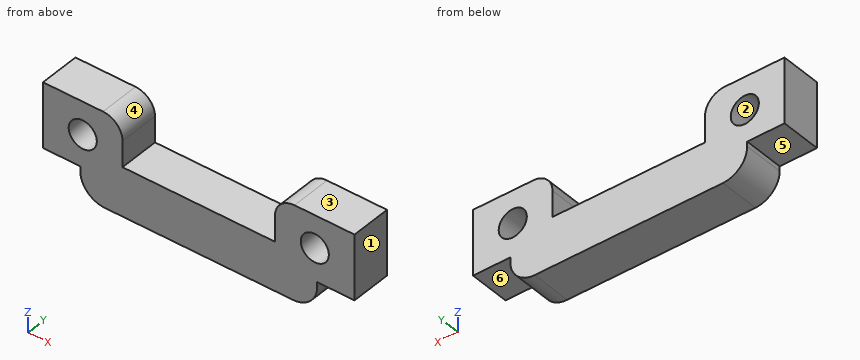
```python
from build123d import *

# Parameters (mm, degrees)
BOSS_EXTRUDE1_DEPTH  = 3.175
M2_CLEARANCE_HOLE1_D = 2.2
SKETCH4_W            = 2.921
SKETCH4_H            = 2.286
CUT_EXTRUDE1_DEPTH   = 4.175
FILLET1_R            = 1.905


with BuildPart() as part:
    # Sketch1 → Boss-Extrude1 (new body)
    with BuildSketch(Plane(origin=(0, 0, 0), x_dir=(1, 0, 0), z_dir=(0, 1, 0))):
        with BuildLine():
            Line((0, -0.127190553), (4.699, -0.127190553))
            ThreePointArc((4.699, -0.127190553), (5.776630735, 0.319178713), (6.223, 1.396809447))
            Line((6.223, 1.396809447), (6.223, 3.428809447))
            Line((6.223, 3.428809447), (18.161, 3.428809447))
            Line((18.161, 3.428809447), (18.161, 1.396809447))
            ThreePointArc((18.161, 1.396809447), (18.607369265, 0.319178713), (19.685, -0.127190553))
            Line((19.685, -0.127190553), (24.384, -0.127190553))
            Line((24.384, -0.127190553), (24.384, 7.238809447))
            Line((24.384, 7.238809447), (0, 7.238809447))
            Line((0, 7.238809447), (0, -0.127190553))
        make_face()
    extrude(amount=BOSS_EXTRUDE1_DEPTH)

    # M2 Clearance Hole1 (through all)
    with Locations(Plane(origin=(0, 0, 0), x_dir=(-1, 0, 0), z_dir=(0, -1, 0))):
        with Locations((-3.1115, 2.412809447), (-21.2725, 2.412809447)):
            Hole(M2_CLEARANCE_HOLE1_D / 2)

    # Sketch4 → Cut-Extrude1 (cut, through all)
    with BuildSketch(Plane.XZ):
        with Locations((22.9235, -6.095809447)):
            Rectangle(SKETCH4_W, SKETCH4_H)
        with Locations((1.4605, -6.095809447)):
            Rectangle(SKETCH4_W, SKETCH4_H)
    extrude(amount=-CUT_EXTRUDE1_DEPTH, mode=Mode.SUBTRACT)

    # Fillet1
    fillet1_edges = [part.edges().sort_by_distance(p)[0] for p in [
        (21.463, 1.5875, -7.238809447),
        (2.921, 1.5875, -7.238809447),
    ]]
    fillet(fillet1_edges, radius=FILLET1_R)


solid = part.part
```
Work out the finished part from the listing and answer in its coordinate system (mm). Face numbers are marked on the shaded views. A direction names the side the tool comes from. Coordinates: 2 decimals unless noted, no trailing zeros. Write each loop counter-clockwise with the first axis right and the second up, starting at its lowest first coordinate (ties: lowest second). Pieces come first, ordered by that corner, then holes.
Q1. Find the intervals of material crossed by line 1 (X direction, y = 2.7, z = -2.5); line 2 (X direction, y = 2.9, z = -3); line 3 (Z direction, x = 7.75, y = 1.95), in increasing order.
Q2. Determine the mould class of the marked faces 1, 2 and 3 for opening direction X: released by +X, released by -X, zero draft, split by the parting line, or undercut.
Q3. A cutting plane is placed at B-B, the plane z = -1. Give the vertices of the cut face in (x, y) (3 decimals), then the cut area to 3 significant figures.
Q4. A cutting plane is placed at A-A, the plane x = 21.25. Give the vertices of the cut face in (y, z) (3 decimals), then the cut area to 3 significant figures.
Q5. Each of these flat-tipped pins is pushed along its axis until it touches: pin 1 Ø1.3 at (x, z) = (3.11, -2.41) entering from +Y; pin 2 Ø1 at (x, y) = (15.5, 1.5) entering from +Z. Where does it stop, or does it pass through?
Q6. A cutting plane is placed at C-C, the plane y = 1.7. State how many separate pieces and enclosed holes the cut face has, then the cut area to 3 significant figures.
Q7. Which of the six approach directions +Z, -Z, +X, -X, +Y, -Y give full straight-line access (tool end or side, diameter ignored) to the marked faces 4, 5 and 6?
Q8. A cutting plane is placed at D-D, the plane x = 16.5. Give the vertices of the cut face in (y, z) (3 decimals), then the cut area to 3 significant figures.
Findings below:
1. line 1: x = 0 to 2.01, 4.21 to 6.22, 18.16 to 20.18, 22.37 to 24.38
1. line 2: x = 0 to 2.18, 4.04 to 6.22, 18.16 to 20.34, 22.2 to 24.38
1. line 3: z = -7.24 to -3.43
2. face 1: released by +X
2. face 2: undercut
2. face 3: zero draft
3. outline: (0, 0) - (6.17, 0) - (6.17, 3.175) - (0, 3.175) - close; (18.214, 0) - (24.384, 0) - (24.384, 3.175) - (18.214, 3.175) - close
3. area: 39.2 mm2
4. outline: (0, -6.209) - (3.175, -6.209) - (3.175, -3.513) - (0, -3.513) - close; (0, -1.313) - (3.175, -1.313) - (3.175, 0.127) - (0, 0.127) - close
4. area: 13.1 mm2
5. pin 1: passes through
5. pin 2: stops at z = -3.43
6. separate pieces: 1
6. enclosed holes: 2
6. area: 114 mm2
7. face 4: +Z, +Y, -Y
7. face 5: -Z, -X, +Y, -Y
7. face 6: -Z, +X, +Y, -Y
8. outline: (0, -7.239) - (3.175, -7.239) - (3.175, -3.429) - (0, -3.429) - close
8. area: 12.1 mm2
